```python
from build123d import *

# Parameters (mm, degrees)
F0_W     = 57.15
F0_H     = 57.15
F0_R     = 1.64973
F0_R_2   = 2.1971
F0_R_3   = 13.97
F1_DEPTH = 9.398
F2_R     = 4.12496
F2_R_2   = 2.1971
F3_DEPTH = 6.35
F4_R     = 13.97
F5_DEPTH = 2.286
F6_R     = 3.81


with BuildPart() as f1:
    # F0 (on Front) → F1 (new body)
    with BuildSketch(Plane.XZ):
        Rectangle(F0_W, F0_H)
        with Locations((-23.495, -23.495)):
            Circle(F0_R, mode=Mode.SUBTRACT)
        with Locations((-14.142107, -14.142107)):
            Circle(F0_R_2, mode=Mode.SUBTRACT)
        with Locations((23.495, -23.495)):
            Circle(F0_R, mode=Mode.SUBTRACT)
        with Locations((14.142107, -14.142107)):
            Circle(F0_R_2, mode=Mode.SUBTRACT)
        with Locations((-14.142107, 14.142107)):
            Circle(F0_R_2, mode=Mode.SUBTRACT)
        with Locations((-23.495, 23.495)):
            Circle(F0_R, mode=Mode.SUBTRACT)
        Circle(F0_R_3, mode=Mode.SUBTRACT)
        with Locations((14.142107, 14.142107)):
            Circle(F0_R_2, mode=Mode.SUBTRACT)
        with Locations((23.495, 23.495)):
            Circle(F0_R, mode=Mode.SUBTRACT)
    extrude(amount=F1_DEPTH)

    # F2 (on face) → F3 (cut)
    with BuildSketch(Plane.XZ.offset(9.398)):
        with Locations((-14.142107, 14.142107)):
            Circle(F2_R)
        with Locations((-14.142107, 14.142107)):
            Circle(F2_R_2, mode=Mode.SUBTRACT)
        with Locations((14.142107, 14.142107)):
            Circle(F2_R)
        with Locations((14.142107, 14.142107)):
            Circle(F2_R_2, mode=Mode.SUBTRACT)
        with Locations((14.142107, -14.142107)):
            Circle(F2_R)
        with Locations((14.142107, -14.142107)):
            Circle(F2_R_2, mode=Mode.SUBTRACT)
        with Locations((-14.142107, -14.142107)):
            Circle(F2_R)
        with Locations((-14.142107, -14.142107)):
            Circle(F2_R_2, mode=Mode.SUBTRACT)
    extrude(amount=-F3_DEPTH, mode=Mode.SUBTRACT)

    # F4 (on face) → F5 (cut)
    with BuildSketch(Plane.XZ.offset(9.398)):
        with BuildLine():
            ThreePointArc((15.99836, -10.458411), (18.318168, -5.456245), (19.1135, 0))
            ThreePointArc((19.1135, 0), (18.318168, 5.456245), (15.99836, 10.458411))
            ThreePointArc((15.99836, 10.458411), (11.22532, 11.22532), (10.458411, 15.99836))
            ThreePointArc((10.458411, 15.99836), (0, 19.1135), (-10.458411, 15.99836))
            ThreePointArc((-10.458411, 15.99836), (-10.128979, 15.096097), (-10.017147, 14.142107))
            ThreePointArc((-10.017147, 14.142107), (-11.97897, 10.629824), (-15.99836, 10.458411))
            ThreePointArc((-15.99836, 10.458411), (-19.1135, 0), (-15.99836, -10.458411))
            ThreePointArc((-15.99836, -10.458411), (-11.97897, -10.629824), (-10.017147, -14.142107))
            ThreePointArc((-10.017147, -14.142107), (-10.128979, -15.096097), (-10.458411, -15.99836))
            ThreePointArc((-10.458411, -15.99836), (0, -19.1135), (10.458411, -15.99836))
            ThreePointArc((10.458411, -15.99836), (11.22532, -11.22532), (15.99836, -10.458411))
        make_face()
        Circle(F4_R, mode=Mode.SUBTRACT)
    extrude(amount=-F5_DEPTH, mode=Mode.SUBTRACT)

    # F6
    f6_edges = [f1.edges().sort_by_distance(p)[0] for p in [
        (-28.575, -4.699, 28.575),
        (28.575, -4.699, 28.575),
        (28.575, -4.699, -28.575),
        (-28.575, -4.699, -28.575),
    ]]
    fillet(f6_edges, radius=F6_R)


solid = f1.part
```
Here's how the part is built. I have some questions about the finished solid (model axes, mm). A direction names the side the tool comes from. Give positions to 0.01 mm unless a question says otherwise; leave off trailing zeros. Order: outer loops, then holes, each group sorted by start corner. A loop starts at its lowest first (then second) coordinate and runs counter-clockwise, first axis right, second up. Notation, with made-up numbers: M -14.75,83 L 20.25,83 A27 cw 20.25,113 Z; hole C 27.25,19 d10. An arc over 180 degrees is marked long. Use a Markdown table: item, result. Add a question column.
1. On a 3-axis mill with a long thin cutter (end or side, diameter ignored), from which of +Z, -Z, +X, -X, +Y, -Y can I reach the whole of each face in a straight line? I mean faces 1 (the flat face through (0, -5, -28.575)), 2 (the cylindrical face through (-17.18, -5.56, 16.93)). Say none if no direction works.
2. Suppose I cut it at A-A (x = 0). List the corners of the cut face in (y, z) for me (1 decimal), and give its area (3 significant figures).
3. I need wall thicknesses on probe 1 along Z at (x, y) = (14, -2.25) (3 decimals); probe 2 along Z at (x, y) = (-23.5, -5) (3 decimals); probe 3 along X at (y, z) = (-5, -17) (3 decimals). Which ranges of each line are inside material? Lowest first, please. Write a range as from..to.
4. For pin 1 Ø4 at (x, z) = (-15, -12.5) entering from -Y; pin 2 Ø3.5 at (x, z) = (-14.14, -14.14) entering from +Y, each with a flat end and sliding along its axis, tell me the tip position at first contact or that it passes through.
5. Suppose I cut it at C-C (y = -8.5). List the corners of the cut face in (x, z) for me (1 decimal).
6. Suppose I cut it at B-B (z = 13). List the corners of the cut face in (x, y) for me (3 decimals).
7. If we mould it in two halves opening along X, with no side actions, what happens to faces 3 (the flat face through (-0.4, -9.398, 19.5)), 4 (the cylindrical face through (27.43, -4.76, 27.49)), 5 (the flat face through (-12, -3.048, 12))? For each: +X half, -X half, draft (parallel to the pull), parting line (faces both ways), or undercut.
8. Suppose I cut it at D-D (y = -4.75). Give the number of separate pieces and of enclosed holes in the cut face, and give its area (3 significant figures).
Results list:
| question | item | result |
|---|---|---|
| 1 | face 1 | -Z, +X, -X, +Y, -Y |
| 1 | face 2 | -Y |
| 2 | outline | M -9.4,-28.6 L 0,-28.6 L 0,-14 L -7.1,-14 L -7.1,-19.1 L -9.4,-19.1 Z; M -9.4,19.1 L -7.1,19.1 L -7.1,14 L 0,14 L 0,28.6 L -9.4,28.6 Z |
| 2 | area | 251 mm² |
| 3 | probe 1 | z = -28.575..-16.335, -11.95..11.95, 16.335..28.575 |
| 3 | probe 2 | z = -28.575..-25.145, -21.845..21.845, 25.145..28.575 |
| 3 | probe 3 | x = -28.575..-17.117, -11.168..11.168, 17.117..28.575 |
| 4 | pin 1 | stops at y = -3.05 |
| 4 | pin 2 | passes through |
| 5 | outline | M -28.6,-24.8 A3.8 ccw -24.8,-28.6 L 24.8,-28.6 A3.8 ccw 28.6,-24.8 L 28.6,24.8 A3.8 ccw 24.8,28.6 L -24.8,28.6 A3.8 ccw -28.6,24.8 Z; hole C -23.5,-23.5 d3.3; hole C -23.5,23.5 d3.3; hole M -16,-10.5 A4.1 ccw long -10.5,-16 A19.1 ccw 10.5,-16 A4.1 ccw long 16,-10.5 A19.1 ccw 19.1,0 A19.1 ccw 16,10.5 A4.1 ccw long 10.5,16 A19.1 ccw -10.5,16 A4.1 ccw long -16,10.5 A19.1 ccw Z; hole C 23.5,-23.5 d3.3; hole C 23.5,23.5 d3.3 |
| 6 | outline | M -28.575,-9.398 L -18.106,-9.398 L -18.106,-3.048 L -16.019,-3.048 L -16.019,0 L -28.575,0 Z; M -12.265,-3.048 L -10.178,-3.048 L -10.178,-7.112 L -5.115,-7.112 L -5.115,0 L -12.265,0 Z; M 5.115,-7.112 L 10.178,-7.112 L 10.178,-3.048 L 12.265,-3.048 L 12.265,0 L 5.115,0 Z; M 16.019,-3.048 L 18.106,-3.048 L 18.106,-9.398 L 28.575,-9.398 L 28.575,0 L 16.019,0 Z |
| 7 | face 3 | draft |
| 7 | face 4 | +X half |
| 7 | face 5 | undercut |
| 8 | separate pieces | 1 |
| 8 | enclosed holes | 9 |
| 8 | area | 2,390 mm² |
